Check sheet for the modelled part. Datum: model origin and axes. Units: mm. A direction names the side the tool comes from. Give positions to 0.01 mm unless a question says otherwise; leave off trailing zeros. Loops run counter-clockwise (first coordinate to the right, second up) from the corner with the lowest first, then second, coordinate; pieces in that order, holes last. Notation, with made-up numbers: (34, 72) - (64, 72) arc R15 ccw to (64, 89) - close; hole circle Ø8 at (-40, 52.25). An arc over 180 degrees is marked (long way). Use one line per item in the form item = value.
from build123d import *

# Parameters (mm, degrees)
DODANIE_WYCI_GNI_CIE1_DEPTH     = 8
SZKIC4_R                        = 3
WYTNIJ_WYCI_GNI_CIE1_DEPTH      = 51.635955605
ZAOKR_GLENIE1_R                 = 1.5
WYTNIJ_WYCI_GNI_CIE4_START      = -16
WYTNIJ_WYCI_GNI_CIE4_DEPTH      = 16
WYTNIJ_WYCI_GNI_CIE8_DEPTH      = 36.191937997
WYTNIJ_WYCI_GNI_CIE8_DEPTH_BACK = 36.191937997
SZKIC15_W                       = 2
SZKIC15_H                       = 6.5
SZKIC16_R                       = 3
DODANIE_WYCI_GNI_CIE2_DEPTH     = 11.5
DODANIE_WYCI_GNI_CIE3_START     = -3
SZKIC17_R                       = 3
DODANIE_WYCI_GNI_CIE3_DEPTH     = 3
OTWORY_USTALAJ_CE_6_0MM1_D      = 6
OTWORY_USTALAJ_CE_6_0MM1_DEPTH  = 1
OTWORY_USTALAJ_CE_6_0MM1_TIP    = 1.802581857


# Read off the part's stored shape, not the designer's step: Wytnij-wyciągnięcie4
with BuildPart() as part:
    # Szkic1 → Dodanie-wyciągnięcie1 (new, symmetric)
    with BuildSketch(Plane.XY):
        with BuildLine():
            ThreePointArc((-16, 0), (0, -16), (16, 0))
            Line((16, 0), (30, 0))
            Line((30, 0), (30, -40))
            Line((30, -40), (-30, -40))
            Line((-30, -40), (-30, 0))
            Line((-30, 0), (-16, 0))
        make_face()
        with BuildLine():
            ThreePointArc((-14, 0), (0, -14), (14, 0))
            Line((14, 0), (16, 0))
            ThreePointArc((16, 0), (0, -16), (-16, 0))
            Line((-16, 0), (-14, 0))
        make_face()
    extrude(amount=DODANIE_WYCI_GNI_CIE1_DEPTH, both=True)

    # Szkic4 → Wytnij-wyciągnięcie1 (cut, through all)
    with BuildSketch(Plane(origin=(0, 0, 0), x_dir=(1, 0, 0), z_dir=(0, 1, 0))):
        with BuildLine():
            ThreePointArc((-18.65, -8), (-26.65, 0), (-18.65, 8))
            Line((-18.65, 8), (-30, 8))
            Line((-30, 8), (-30, -8))
            Line((-30, -8), (-18.65, -8))
        make_face()
        with BuildLine():
            Line((30, 8), (18.65, 8))
            ThreePointArc((18.65, 8), (26.65, 0), (18.65, -8))
            Line((18.65, -8), (30, -8))
            Line((30, -8), (30, 8))
        make_face()
        with Locations(Location((21.4, 0, 0), (0, 0, 270))):
            Circle(SZKIC4_R)
        with Locations(Location((-21.4, 0, 0), (0, 0, 270))):
            Circle(SZKIC4_R)
    extrude(amount=-WYTNIJ_WYCI_GNI_CIE1_DEPTH, mode=Mode.SUBTRACT)

    # Zaokrąglenie1
    zaokr_glenie1_edges = [part.edges().sort_by_distance(p)[0] for p in [
        (0, -14, 8),
    ]]
    fillet(zaokr_glenie1_edges, radius=ZAOKR_GLENIE1_R)

    # Wytnij-wyciągnięcie4 outline → Wytnij-wyciągnięcie4 (cut)
    with BuildSketch(Plane(origin=(0, 0, -8), x_dir=(-1, 0, 0), z_dir=(0, 0, -1)).offset(WYTNIJ_WYCI_GNI_CIE4_START)):
        Polygon((-16, -16.5), (-16, -5), (-37.876810691, -5), (-37.876810691, -40), (49.702662137, -40), (49.702662137, -5), (16, -5), (16, -16.5), align=None)
    extrude(amount=WYTNIJ_WYCI_GNI_CIE4_DEPTH, mode=Mode.SUBTRACT)

    # Szkic15 → Wytnij-wyciągnięcie8 (cut, two sides: drawn at the far end of the back side and taken through both)
    with BuildSketch(Plane.XY.offset(8).offset(-WYTNIJ_WYCI_GNI_CIE8_DEPTH_BACK)):
        with Locations((15, -13.25)):
            Rectangle(SZKIC15_W, SZKIC15_H)
        with Locations((-15, -13.25)):
            Rectangle(SZKIC15_W, SZKIC15_H)
    extrude(amount=WYTNIJ_WYCI_GNI_CIE8_DEPTH + WYTNIJ_WYCI_GNI_CIE8_DEPTH_BACK, mode=Mode.SUBTRACT)

    # Szkic16 → Dodanie-wyciągnięcie2 (add)
    # profile 1 of 2: a face of its own
    with BuildSketch(Plane.XZ.offset(5)):
        with BuildLine():
            Line((-16, 8), (-16, -8))
            Line((-16, -8), (-18.65, -8))
            ThreePointArc((-18.65, -8), (-26.65, 0), (-18.65, 8))
            Line((-18.65, 8), (-16, 8))
        make_face()
        with Locations(Location((-21.4, 0, 0), (0, 0, 90))):
            Circle(SZKIC16_R, mode=Mode.SUBTRACT)
    # profile 2 of 2: a face of its own
    with BuildSketch(Plane.XZ.offset(5)):
        with BuildLine():
            Line((16, 8), (16, -8))
            Line((16, -8), (18.65, -8))
            ThreePointArc((18.65, -8), (26.65, 0), (18.65, 8))
            Line((18.65, 8), (16, 8))
        make_face()
        with Locations(Location((21.4, 0, 0), (0, 0, 90))):
            Circle(SZKIC16_R, mode=Mode.SUBTRACT)
    extrude(amount=DODANIE_WYCI_GNI_CIE2_DEPTH)

    # Szkic17 → Dodanie-wyciągnięcie3 (add)
    with BuildSketch(Plane.XZ.offset(16.5).offset(DODANIE_WYCI_GNI_CIE3_START)):
        with Locations(Location((-21.4, 0, 0), (0, 0, 90))):
            Circle(SZKIC17_R)
        with Locations(Location((21.4, 0, 0), (0, 0, 90))):
            Circle(SZKIC17_R)
    extrude(amount=DODANIE_WYCI_GNI_CIE3_DEPTH)

    # Otwory ustalające Ø6.0mm1
    with Locations(Plane(origin=(-21.4, -13.5, 0), x_dir=(0, 0, 1), z_dir=(0, 1, 0))):
        with Locations((0, 0), (0, 42.8)):
            Hole(OTWORY_USTALAJ_CE_6_0MM1_D / 2, depth=OTWORY_USTALAJ_CE_6_0MM1_DEPTH)
            with Locations((0, 0, -(OTWORY_USTALAJ_CE_6_0MM1_DEPTH + OTWORY_USTALAJ_CE_6_0MM1_TIP / 2))):  # 118° drill point
                Cone(0, OTWORY_USTALAJ_CE_6_0MM1_D / 2, OTWORY_USTALAJ_CE_6_0MM1_TIP, mode=Mode.SUBTRACT)


solid = part.part
Item 1: Thickness scan on L1, parallel to X at y = -12.75, z = 5.75; L2, parallel to X at y = -8.75, z = 0; L3, parallel to X at y = -11.25, z = 0. Record the ranges inside material, lowest first.
Answer block:
L1 = -24.21 to -16, -14 to -5.78, 5.78 to 14, 16 to 24.21
L2 = -26.65 to -24.4, -18.4 to -10.93, 10.93 to 18.4, 24.4 to 26.65
L3 = -26.65 to -24.4, -18.4 to -16, -14 to -8.33, 8.33 to 14, 16 to 18.4, 24.4 to 26.65
Item 2: Access from +Z, -Z, +X, -X, +Y, -Y to the whole of each face (thin tool, end or side, straight path). Record for faces 1 (the face through (-24.393, -7.148, 0.198)), 2 (the face through (-14, -13, 0)), 3 (the face through (-4.4, -15.5, 8)).
Answer block:
face_1 = +Y
face_2 = +Z, -Z, -Y
face_3 = +Z, +X, -X, +Y, -Y
Item 3: Section check C-C on y = -15. Give the number of separate pieces and of enclosed holes in the cut face, then the cut area to 3 significant figures.
Answer block:
separate_pieces = 3
enclosed_holes = 2
area = 704 mm2
Item 4: Section check B-B on z = 5.75. Record the boundary of the cut face in (x, y).
Answer block:
outline = (-24.21, -16.5) - (-16, -16.5) - (-16, -10) - (-14, -10) - (-14, -16.5) - (14, -16.5) - (14, -10) - (16, -10) - (16, -16.5) - (24.21, -16.5) - (24.21, 0) - (14, 0) arc R14 cw to (-14, 0) - (-24.21, 0) - close
Item 5: Gauge pin test, flat ends, axial feed: P1, Ø1, axis at x = -15, z = 0, coming from the -Y side; P2, Ø2, axis at y = -11.5, z = 5, coming from the -X side; P3, Ø3, axis at y = -12.5, z = -4, coming from the -X side. Record the tip position at first contact, or that the pin passes through.
Answer block:
P1 = -10
P2 = -25.58
P3 = -26.25
Item 6: Mould release check, pull along X, two halves, no side actions. Record for faces 4 (the face through (-26.648, -8.134, -0.176)), 5 (the face through (0, -16.5, 0)), 6 (the face through (14, -13, 0)): released by +X, released by -X, zero draft, split by the parting line, or undercut.
Answer block:
face_4 = released by -X
face_5 = zero draft
face_6 = undercut
Item 7: Section check A-A on x = 0. Record the boundary of the cut face in (y, z).
Answer block:
outline = (-16.5, -8) - (-14, -8) - (-14, 6.5) arc R1.5 ccw to (-15.5, 8) - (-16.5, 8) - close
